Can you work these out from the drawing? Everything is in mm from the part's minimum corner. A direction names the side the tool comes from. Coordinates: 2 decimals unless noted, no trailing zeros. Loops run counter-clockwise (first coordinate to the right, second up) from the corner with the lowest first, then second, coordinate; pieces in that order, holes last.
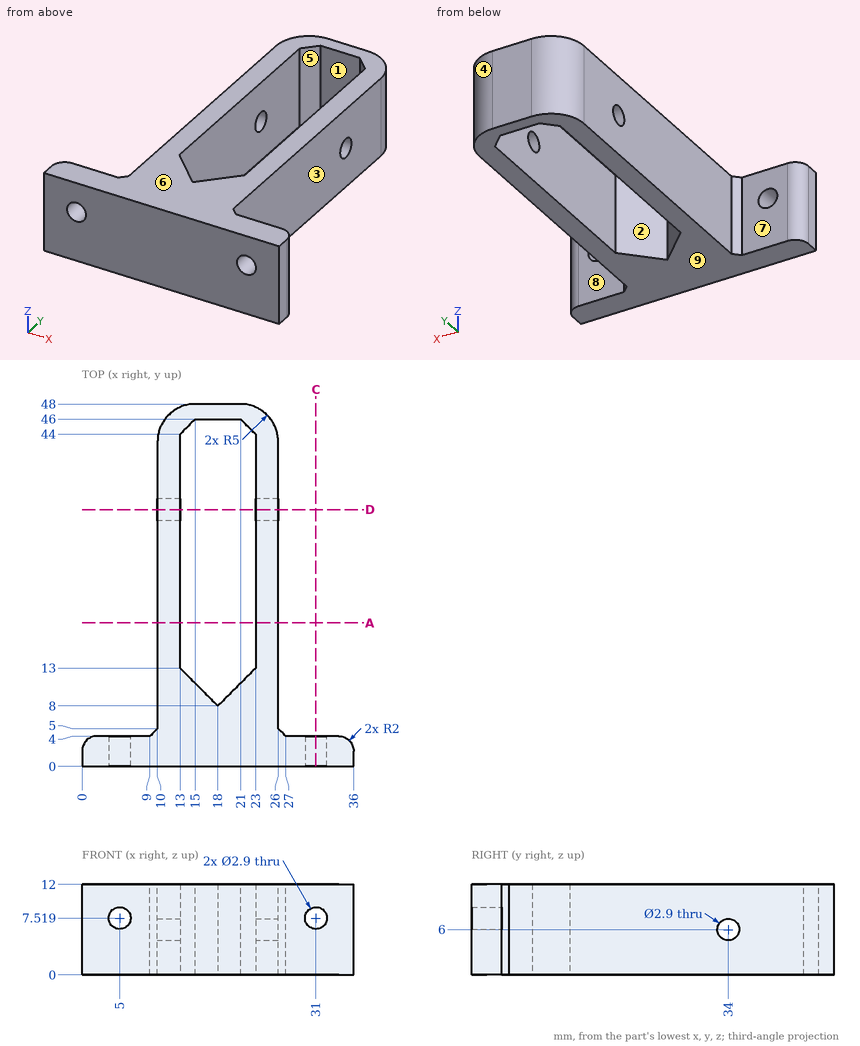
1) For the marked faces 5, 6, 7, 8 and 9, which set-ups out of +Z, -Z, +X, -X, +Y, -Y let a thin tool reach every point of the face, with its end or its side?
2) We'd pull the mould along Y, two halves only. Please class the marked faces 1, 2, 3 and 4: released by +Y, released by -Y, zero draft, split by the parting line, or undercut.
3) Imagine slicing it at A-A on y = 19. List the corners of the cut face in (x, z) for me.
4) Imagine slicing it at C-C on x = 31. List the corners of the cut face in (y, z) for me.
5) Will these pins go through, and if not, where does the flat tip stop? pin 1 (6 mm diameter, centred on y = 39, z = 9.5, fed in from +X); pin 2 (3.5 mm diameter, centred on y = 34, z = 6, fed in from -X); pin 3 (2 mm diameter, centred on x = 6, z = 3.5, fed in from +Y).
6) If I drill on L1, parallel to X at y = 35, z = 1.75; L2, parallel to Y at x = 17, z = 7.75; L3, parallel to Z at x = 5, y = 1.6, over which ranges is the centre line in solid material (lowest first)?
7) Imagine slicing it at D-D on y = 34. List the corners of the cut face in (x, z) for me, plus the area to 3 significant figures.
Solved:
1. face 5: +Z, -Z
1. face 6: +Z, +X, -X, +Y, -Y
1. face 7: +Z, -Z, -X, +Y
1. face 8: +Z, -Z, +X, +Y
1. face 9: -Z, +X, -X, +Y, -Y
2. face 1: undercut
2. face 2: undercut
2. face 3: zero draft
2. face 4: released by +Y
3. outline: (10, 0) - (13, 0) - (13, 12) - (10, 12) - close; (23, 0) - (26, 0) - (26, 12) - (23, 12) - close
4. outline: (0, 0) - (4, 0) - (4, 6.07) - (0, 6.07) - close; (0, 8.97) - (4, 8.97) - (4, 12) - (0, 12) - close
5. pin 1: stops at x = 26
5. pin 2: stops at x = 10
5. pin 3: stops at y = 4
6. L1: x = 10 to 13, 23 to 26
6. L2: y = 0 to 9, 46 to 48
6. L3: z = 0 to 6.07, 8.97 to 12
7. outline: (10, 0) - (13, 0) - (13, 4.55) - (10, 4.55) - close; (10, 7.45) - (13, 7.45) - (13, 12) - (10, 12) - close; (23, 0) - (26, 0) - (26, 4.55) - (23, 4.55) - close; (23, 7.45) - (26, 7.45) - (26, 12) - (23, 12) - close
7. area: 54.6 mm2
